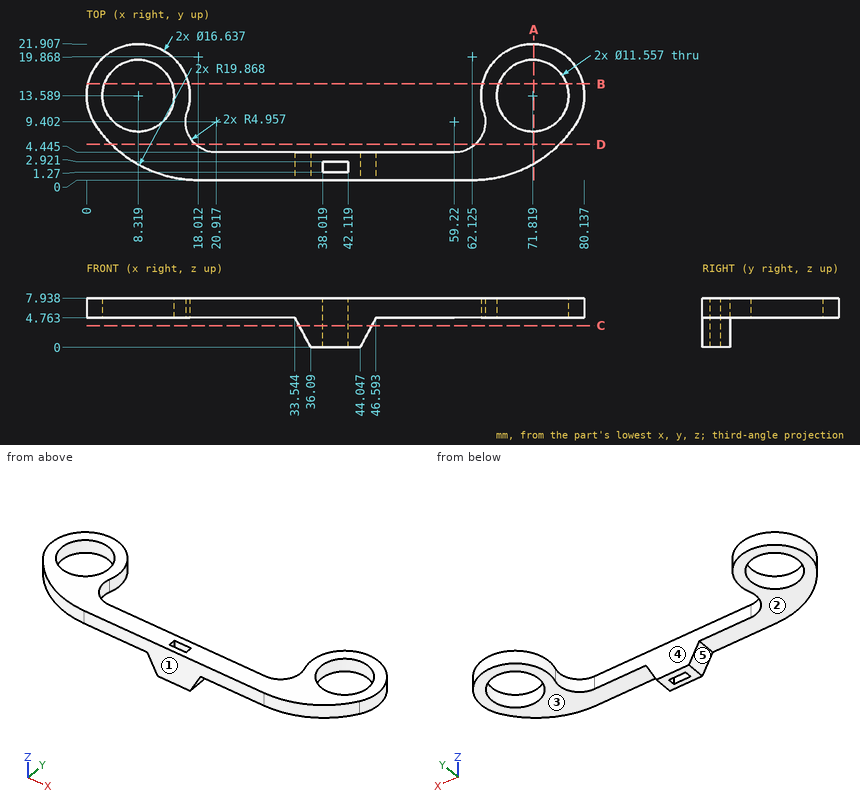
Input: dimensioned drawing with shaded views. Units: mm. Origin: part minimum x, y, z. A direction names the side the tool comes from. Coordinates: 2 decimals unless noted, no trailing zeros. Write each loop counter-clockwise with the first axis right and the second up, starting at its lowest first coordinate (ties: lowest second). Pieces come first, ordered by that corner, then holes. Notation, with made-up numbers: (14.5, 11.25) -> (23.5, 11.25) arc R16 cw to (23.5, 32.25) -> close; hole circle Ø10 at (67, 19). An arc over 180 degrees is marked (long way). Return JSON: item names as keys, results as strings. Group by question number.
1) Section query C-C, the plane z = 3.5. Return loops of the section in (x, y) (1 decimal).
2) Ray query, line 1 along X through (y, z) = (9, 6.5) (1 decimal); line 2 along Y through (x, z) = (51, 6.75) (1 decimal); line 3 along X through (y, z) = (6.75, 7.75) (1 decimal). Return the intervals inside material, ascending.
3) Section query A-A, the plane x = 72. Return loops of the section in (y, z) (1 decimal).
4) Set-up query: the marked faces 1 and 2. Return all of +Z, -Z, +X, -X, +Y, -Y with unobstructed straight access to the full face (end or side cutting, diameter ignored); none if empty.
5) Section query D-D, the plane y = 5.75. Return loops of the section in (x, z) (1 decimal).
6) Contact query for flat-ended pins moving along their axis: P1, Ø0.8, axis at y = 2, z = 6, coming from the -X side (1 decimal); P2, Ø3.5, axis at x = 39.5, z = 2.5, coming from the +Y side (1 decimal); P3, Ø5, axis at x = 66, y = 18.5, coming from the -Z side; P4, Ø2, axis at y = 13.5, z = 3, coming from the -X side. Output: stop coordinate, or through.
7) Section query B-B, the plane y = 15.5. Return loops of the section in (x, z) (1 decimal).
8) Mould query, pull axis X, two halves, no side actions, for the marked faces 3, 4 and 5. Classes: +X half, -X half, draft (parallel to the pull), parting line (faces both ways), or undercut.
From the geometry:
{
 "1": {"outline": "(34.2, 0) -> (45.9, 0) -> (45.9, 4.4) -> (34.2, 4.4) -> close; hole (38, 1.3) -> (42.1, 1.3) -> (42.1, 2.9) -> (38, 2.9) -> close"},
 "2": {"line 1": "1.4 to 4.8, 11.8 to 16, 64.2 to 68.3, 75.3 to 78.8", "line 2": "0 to 4.4", "line 3": "3.1 to 16.7, 63.4 to 77"},
 "3": {"outline": "(2.6, 4.8) -> (7.8, 4.8) -> (7.8, 7.9) -> (2.6, 7.9) -> close; (19.4, 4.8) -> (21.9, 4.8) -> (21.9, 7.9) -> (19.4, 7.9) -> close"},
 "4": {"face 1": "+Z, -Z, +X, -X, -Y", "face 2": "-Z, -X, +Y, -Y"},
 "5": {"outline": "(4, 4.8) -> (17.6, 4.8) -> (17.6, 7.9) -> (4, 7.9) -> close; (62.6, 4.8) -> (76.1, 4.8) -> (76.1, 7.9) -> (62.6, 7.9) -> close"},
 "6": {"P1": "x = 8.5", "P2": "y = 4.4", "P3": "z = 4.76", "P4": "through"},
 "7": {"outline": "(0.2, 4.8) -> (2.9, 4.8) -> (2.9, 7.9) -> (0.2, 7.9) -> close; (13.8, 4.8) -> (16.4, 4.8) -> (16.4, 7.9) -> (13.8, 7.9) -> close; (63.7, 4.8) -> (66.4, 4.8) -> (66.4, 7.9) -> (63.7, 7.9) -> close; (77.3, 4.8) -> (79.9, 4.8) -> (79.9, 7.9) -> (77.3, 7.9) -> close"},
 "8": {"face 3": "draft", "face 4": "undercut", "face 5": "-X half"}
}
